```python
from build123d import *

# Parameters (mm, degrees)
BOSS_EXTRUDE5_START      = -4.7625
BOSS_EXTRUDE5_DEPTH      = 9.525
SKETCH6_R                = 1.778
CUT_EXTRUDE3_DEPTH       = 504.733086563
CUT_EXTRUDE4_START       = 3.556
SKETCH7_R                = 3.048
SKETCH7_R_2              = 1.778
CUT_EXTRUDE4_DEPTH       = 505.502600354
CUT_EXTRUDE5_DEPTH       = 506.075936751
SKETCH10_R               = 1.778
CUT_EXTRUDE6_DEPTH       = 502.305599398
CUT_EXTRUDE11_DEPTH      = 3.556
CUT_EXTRUDE11_DEPTH_BACK = 498.926861427
SKETCH12_R               = 3.048
SKETCH13_R               = 1.778
CUT_EXTRUDE12_DEPTH      = 500.236768439
CUT_EXTRUDE13_DEPTH      = 3.556
CUT_EXTRUDE13_DEPTH_BACK = 497.703321125
SKETCH14_R               = 3.048


# Read off the part's stored shape, not the designer's step: Boss-Extrude5
with BuildPart() as part:
    # Boss-Extrude5 outline → Boss-Extrude5 (new body)
    with BuildSketch(Plane(origin=(0, 0, 4.097149242), x_dir=(-1, 0, 0), z_dir=(0, 0, -1)).offset(BOSS_EXTRUDE5_START)):
        with BuildLine():
            add(Edge.make_bspline(
                [(398.35171036, -68.196818162), (396.265786035, -68.16801087), (352.35609282, -67.485074441), (308.459309619, -65.190615284), (266.801551376, -61.551589611)],
                knots=[0.388247103, 0.388247103, 0.388247103, 0.388247103, 0.401472843, 0.666666775, 0.666666775, 0.666666775, 0.666666775], degree=3))
            ThreePointArc((398.35171036, -68.196818162), (445.202941044, -75.692238551), (487.961522574, -96.257326662))
            ThreePointArc((487.961522574, -96.257326662), (494.102034598, -94.922101367), (492.499924864, -88.845757162))
            ThreePointArc((492.499924864, -88.845757162), (472.347982204, -65.669309605), (471.824439099, -34.961421092))
            ThreePointArc((471.824439099, -34.961421092), (471.408544547, -32.082865726), (468.823110549, -30.750731982))
            Line((468.823110549, -30.750731982), (459.298110549, -30.750731982))
            ThreePointArc((459.298110549, -30.750731982), (456.664489609, -32.15241144), (456.356218194, -35.119840174))
            ThreePointArc((456.356218194, -35.119840174), (459.13228847, -45.417631787), (459.332762362, -56.081162557))
            ThreePointArc((459.332762362, -56.081162557), (457.466080229, -59.75328384), (453.620807302, -61.230731982))
            Line((453.620807302, -61.230731982), (423.379813153, -61.230732209))
            add(Edge.make_bspline(
                [(384.696694825, -60.817291125), (385.490946956, -60.834366335), (398.383584309, -61.102948796), (411.282715888, -61.232192999), (423.379813153, -61.230732209)],
                knots=[0.584578014, 0.584578014, 0.584578014, 0.584578014, 0.589634714, 0.666658831, 0.666658831, 0.666658831, 0.666658831], degree=3))
            ThreePointArc((384.696694825, -60.817291125), (381.405012252, -59.519394589), (379.749008052, -56.392517605))
            ThreePointArc((379.749008052, -56.392517605), (379.962938882, -45.344267983), (383.481055682, -34.868942675))
            ThreePointArc((383.481055682, -34.868942675), (383.390574332, -31.793909155), (380.736068027, -30.23904122))
            add(Edge.make_bspline(
                [(371.231646974, -29.984054972), (374.399550345, -30.077611409), (377.567706075, -30.162607104), (380.736068027, -30.23904122)],
                knots=[0.554089987, 0.554089987, 0.554089987, 0.554089987, 0.574612442, 0.574612442, 0.574612442, 0.574612442], degree=3))
            ThreePointArc((371.231646974, -29.984054972), (368.497590253, -31.39435755), (368.242362699, -34.460116724))
            ThreePointArc((368.242362699, -34.460116724), (371.193755258, -45.109007009), (370.814996268, -56.152834373))
            ThreePointArc((370.814996268, -56.152834373), (368.993717887, -59.186422189), (365.637179769, -60.305958601))
            add(Edge.make_bspline(
                [(301.916083239, -57.118764264), (304.793492849, -57.314159562), (316.447125042, -58.077219349), (336.889920622, -59.214945623), (355.259103136, -59.965814652), (364.843153704, -60.280423032), (365.637179769, -60.305958601)],
                knots=[0.408750601, 0.408750601, 0.408750601, 0.408750601, 0.427107919, 0.483087827, 0.539067736, 0.544124431, 0.544124431, 0.544124431, 0.544124431], degree=3))
            ThreePointArc((301.916083239, -57.118764264), (297.703900514, -55.115863145), (295.996304567, -50.7755622))
            ThreePointArc((295.996304567, -50.7755622), (297.395526272, -40.599539879), (301.466201974, -31.168800195))
            ThreePointArc((301.466201974, -31.168800195), (301.565948035, -28.066269557), (298.971867926, -26.361454603))
            add(Edge.make_bspline(
                [(289.489598636, -25.664595471), (292.649719638, -25.90542225), (295.810491414, -26.137709697), (298.971867926, -26.361454603)],
                knots=[0.377389823, 0.377389823, 0.377389823, 0.377389823, 0.397912285, 0.397912285, 0.397912285, 0.397912285], degree=3))
            ThreePointArc((289.489598636, -25.664595471), (286.640803233, -27.018955044), (286.365734252, -30.161288915))
            ThreePointArc((286.365734252, -30.161288915), (289.309950073, -39.618561112), (289.709550194, -49.515465879))
            ThreePointArc((289.709550194, -49.515465879), (287.468803622, -53.805389908), (282.855937937, -55.270266537))
            Line((282.855937937, -55.270266537), (268.113256948, -54.036580381))
            add(Edge.make_bspline(
                [(268.113256948, -54.036580381), (262.634745624, -53.56111419), (251.663313863, -52.628696852), (229.81175043, -50.89541865), (191.471827261, -48.203857237), (136.679597141, -45.286916485), (81.835702382, -43.641470214), (43.402846546, -43.138474088), (21.480818831, -43.050269737), (10.476996172, -43.067138198), (4.980483945, -43.087244707)],
                knots=[-0.002434158, -0.002434158, -0.002434158, -0.002434158, 0.060213256, 0.12286067, 0.248155497, 0.498745152, 0.749334808, 0.874629635, 0.937277049, 0.999924463, 0.999924463, 0.999924463, 0.999924463], degree=3))
            Line((4.980483945, -43.087244707), (5.013364858, -50.687454907))
            add(Edge.make_bspline(
                [(266.801551376, -61.551589611), (261.350884009, -61.078554924), (250.433518448, -60.153958667), (228.701217873, -58.434486699), (190.548987698, -55.763104255), (136.042529388, -52.86929541), (81.4824687, -51.236835025), (43.240954482, -50.737883821), (21.43842692, -50.650632415), (10.483916541, -50.667450636), (5.013364858, -50.687454907)],
                knots=[4.0417e-05, 4.0417e-05, 4.0417e-05, 4.0417e-05, 0.062531963, 0.125023508, 0.2500066, 0.499972783, 0.749938966, 0.874922057, 0.937413603, 0.999905149, 0.999905149, 0.999905149, 0.999905149], degree=3))
        make_face()
    boss_extrude5 = extrude(amount=BOSS_EXTRUDE5_DEPTH)

    # Sketch6 → Cut-Extrude3 (cut, through all)
    with BuildSketch(Plane(origin=(0.32087569, -4.366204823, 0), x_dir=(0.9973104440526221, 0.07329309778936742, 0), z_dir=(-0.07329309778936742, 0.9973104440526221, 0))):
        with Locations(Location((-295.34595845, -4.097149242, 0), (0, 0, 180))):
            Circle(SKETCH6_R)
    cut_extrude3 = extrude(amount=-CUT_EXTRUDE3_DEPTH, mode=Mode.SUBTRACT)

    # Sketch7 → Cut-Extrude4 (cut)
    with BuildSketch(Plane(origin=(3.065947832, -41.718823267, 0), x_dir=(-0.9946544730103679, -0.07309790847145088, 0.07293267510222654), z_dir=(-0.07329309778936742, 0.9973104440526221, 0)).offset(CUT_EXTRUDE4_START)):
        with Locations(Location((294.858228733, -17.454132845, 0), (0, 0, 355.817552062))):
            Circle(SKETCH7_R)
        with Locations(Location((294.858228733, -17.454132845, 0), (0, 0, 355.817552062))):
            Circle(SKETCH7_R_2, mode=Mode.SUBTRACT)
    cut_extrude4 = extrude(amount=-CUT_EXTRUDE4_DEPTH, mode=Mode.SUBTRACT)

    # Mirror4: Boss-Extrude5, Cut-Extrude3, Cut-Extrude4 across plane
    add(boss_extrude5.mirror(Plane(origin=(-4.793985166, 0.020740296, 8.859649242), x_dir=(0, 0, 1), z_dir=(-0.9999906416249494, 0.004326275825933448, 0))))
    add(cut_extrude3.mirror(Plane(origin=(-4.793985166, 0.020740296, 8.859649242), x_dir=(0, 0, 1), z_dir=(-0.9999906416249494, 0.004326275825933448, 0))), mode=Mode.SUBTRACT)
    add(cut_extrude4.mirror(Plane(origin=(-4.793985166, 0.020740296, 8.859649242), x_dir=(0, 0, 1), z_dir=(-0.9999906416249494, 0.004326275825933448, 0))), mode=Mode.SUBTRACT)

    # Sketch9 → Cut-Extrude5 (cut, through all)
    with BuildSketch(Plane(origin=(0, 0, -0.665350758), x_dir=(-1, 0, 0), z_dir=(0, 0, -1))):
        Polygon((268.113256948, -54.036580381), (282.855937937, -55.270266537), (282.538222795, -59.066996326), (267.795541806, -57.83331017), (267.467078991, -61.609602167), (-501.730233012, -147.179806135), (-501.730233012, -16.830462442), (271.226711866, -16.830462442), align=None)
    extrude(amount=-CUT_EXTRUDE5_DEPTH, mode=Mode.SUBTRACT)

    # Sketch10 → Cut-Extrude6 (cut, through all)
    with BuildSketch(Plane(origin=(0.536837032, -20.010173799, 0), x_dir=(0.999640317874878, 0.026818554752505906, 0), z_dir=(-0.026818554752505906, 0.999640317874878, 0))):
        with Locations(Location((-376.656171029, -4.097149242, 0), (0, 0, 180))):
            Circle(SKETCH10_R)
    extrude(amount=-CUT_EXTRUDE6_DEPTH, mode=Mode.SUBTRACT)

    # Sketch12 → Cut-Extrude11 (cut, two sides: drawn at the far end of the back side and taken through both)
    with BuildSketch(Plane(origin=(1.545827279, -57.619483473, 0), x_dir=(0.999640317874878, 0.02681855475250591, 0), z_dir=(-0.02681855475250591, 0.999640317874878, 0)).offset(-CUT_EXTRUDE11_DEPTH_BACK)):
        with Locations(Location((-376.656171029, -4.097149242, 0), (0, 0, 180))):
            Circle(SKETCH12_R)
    extrude(amount=CUT_EXTRUDE11_DEPTH + CUT_EXTRUDE11_DEPTH_BACK, mode=Mode.SUBTRACT)

    # Sketch13 → Cut-Extrude12 (cut, through all)
    with BuildSketch(Plane(origin=(0, -30.750731982, 0), x_dir=(1, 0, 0), z_dir=(0, 1, 0))):
        with Locations(Location((-464.060610549, -4.097149242, 0), (0, 0, 270))):
            Circle(SKETCH13_R)
    extrude(amount=-CUT_EXTRUDE12_DEPTH, mode=Mode.SUBTRACT)

    # Sketch14 → Cut-Extrude13 (cut, two sides: drawn at the far end of the back side and taken through both)
    with BuildSketch(Plane(origin=(0, -68.850731982, 0), x_dir=(1, 0, 0), z_dir=(0, 1, 0)).offset(-CUT_EXTRUDE13_DEPTH_BACK)):
        with Locations(Location((-464.060610549, -4.097149242, 0), (0, 0, 270))):
            Circle(SKETCH14_R)
    extrude(amount=CUT_EXTRUDE13_DEPTH + CUT_EXTRUDE13_DEPTH_BACK, mode=Mode.SUBTRACT)


solid = part.part
```
Geometry check sheet. Reference: the model listing, model coordinates, mm. A direction names the side the tool comes from. Coordinates: 2 decimals unless noted, no trailing zeros. Order: outer loops, then holes, each group sorted by start corner. A loop starts at its lowest first (then second) coordinate and runs counter-clockwise, first axis right, second up.
Q1. Draft check along Z on faces 4 (the face through (-388.8, -61.2, -0.665)), 5 (the face through (-472.51, -66.08, 4.16)), 6 (the face through (-374.12, -46.87, 3.02)). Enter one of: released by +Z, released by -Z, zero draft, split by the parting line, or undercut.
Reply:
face 4: released by -Z
face 5: zero draft
face 6: undercut
Q2. Depth check by flat-ended pin: pin 1 Ø2 at (x, z) = (-464.06, 4.1) entering from -Y; pin 2 Ø5 at (y, z) = (-57, 7.5) entering from -X; pin 3 Ø4 at (x, z) = (-319.5, 2) entering from -Y; pin 4 Ø3 at (x, z) = (-437, 4) entering from +Y. Enter the tip coordinate at first touch or a pass-through.
Reply:
pin 1: passes through
pin 2: stops at x = -470.48
pin 3: stops at y = -65.49
pin 4: stops at y = -61.23
Q3. Tool access check on faces 1 (the face through (-462, -30.751, 4)), 2 (the face through (-297.357, -40.739, 4.164)), 3 (the face through (-275.27, -58.46, 4.03)). Record the directions out of +Z, -Z, +X, -X, +Y, -Y that give a thin tool (end or side, any length) a straight path to the whole face; none if there is none.
Reply:
face 1: +Z, -Z, -X, +Y
face 2: +Z, -Z
face 3: +Z, -Z, +Y
Q4. Thickness scan on probe 1 along X at (y, z) = (-37.5, 0); probe 2 along X at (y, z) = (-35.5, 3.25); probe 3 along X at (y, z) = (-41.5, 1). Record the ranges inside material, lowest first.
Reply:
probe 1: x = -471.03 to -457.24, -382.25 to -369.45, -298.41 to -288.88
probe 2: x = -471.64 to -465.62, -462.5 to -456.51, -383.16 to -377.4, -374.28 to -368.69, -299.22 to -295.1, -291.97 to -288.36
probe 3: x = -470.11 to -458.39, -380.85 to -370.58, -297.16 to -289.59
Q5. Sectioned sample at C-C on y = -86.5. Record the cut outline in (x, z).
Reply:
outline: (-488.72, -0.67) - (-471.49, -0.67) - (-471.49, 8.86) - (-488.72, 8.86) - close
Q6. Sectioned sample at A-A on y = -39. Give the number of separate pieces and of enclosed holes in the cut face, and give its area (3 significant figures).
Reply:
separate pieces: 3
enclosed holes: 3
area: 288 mm2
Q7. Sectioned sample at B-B on x = -425.5. Record the cut outline in (y, z).
Reply:
outline: (-70.84, -0.67) - (-61.23, -0.67) - (-61.23, 8.86) - (-70.84, 8.86) - close
